Part print with two shaded views. Sizes in mm from the minimum x, y, z corner. Round coordinates to 2 decimals unless told otherwise and drop trailing zeros. Loops run counter-clockwise (first coordinate to the right, second up) from the corner with the lowest first, then second, coordinate; pieces in that order, holes last. Notation, with made-up numbers: (88.5, 24.5) -> (127.5, 24.5) arc R13 ccw to (127.5, 43.5) -> close; hole circle Ø6 at (23, 53). An arc over 180 degrees is marked (long way). Use a Markdown table: item, result. Add a question column.
Item 1: Flat gauge pins, fed straight in: pin 1 (10 mm diameter, centred on y = 6.5, z = 28, fed in from +X); pin 2 (1.5 mm diameter, centred on y = 26.5, z = 34, fed in from +X) (1 decimal). Where does each tip first touch, or does it go through?
Item 2: Cut at C-C, the plane y = 9.5. List the corners of the cut face in (x, z).
Item 3: Cut at D-D, the plane z = 17. List the corners of the cut face in (x, y) (1 decimal).
Item 4: Two-plate mould, pull along X, no slides. Class the marked faces 1, 2 and 3: pulls with the +X half, pulls with the -X half, needs draft (parallel to the pull), parting line crosses it, or undercut.
Item 5: Cut at B-B, the plane x = 23. List the corners of the cut face in (y, z) (1 decimal).
Item 6: Probe line 1 (Z direction, x = 15.5, y = 13); line 2 (X direction, y = 22, z = 22) (1 decimal); line 3 (X direction, y = 8, z = 22). List the from-to ranges inside material, lowest first. Write a range as [from, to].
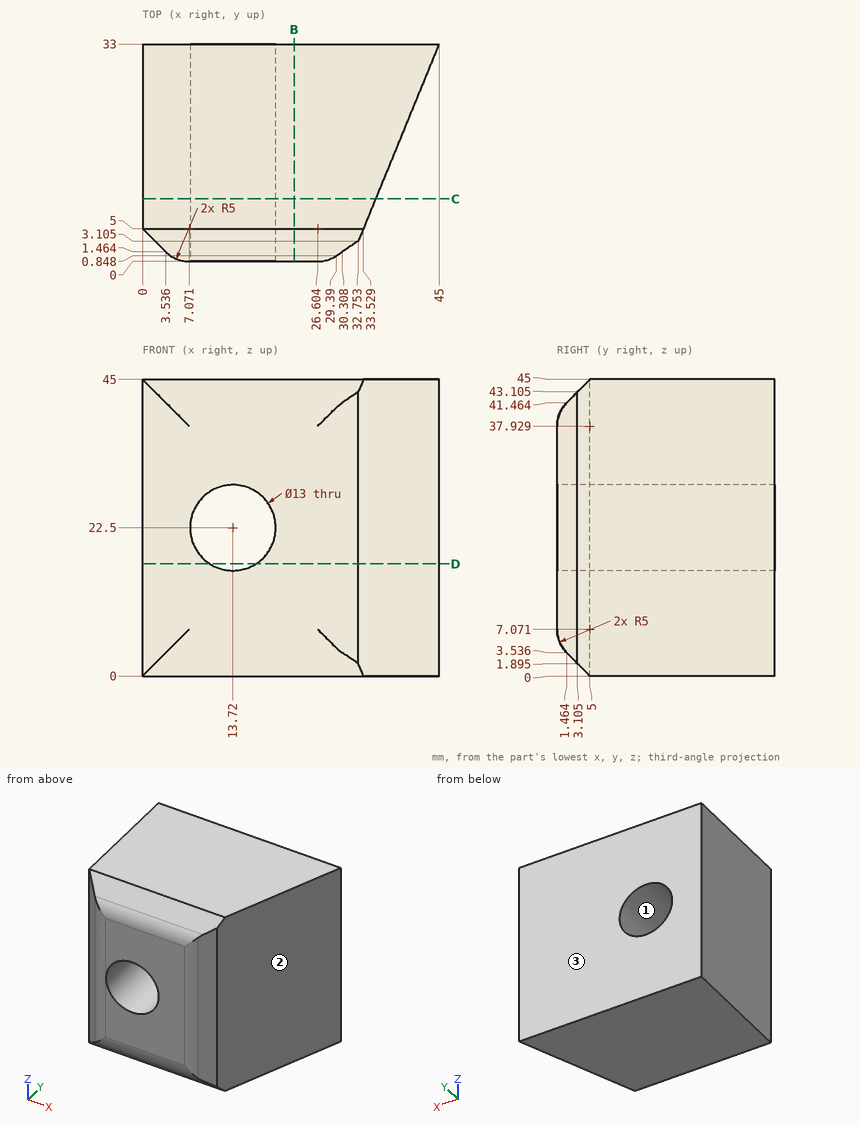
A:
| question | item | result |
|---|---|---|
| 1 | pin 1 | stops at x = 36.19 |
| 1 | pin 2 | stops at x = 42.6 |
| 2 | outline | (0, 0) -> (35.37, 0) -> (35.37, 45) -> (0, 45) -> close; hole circle Ø13 at (13.72, 22.5) |
| 3 | outline | (0, 5) -> (3.5, 1.5) arc R5 ccw to (7.1, 0) -> (10.3, 0) -> (10.3, 33) -> (0, 33) -> close; (17.2, 0) -> (26.6, 0) arc R5 ccw to (29.4, 0.8) -> (32.8, 3.1) -> (45, 33) -> (17.2, 33) -> close |
| 4 | face 1 | undercut |
| 4 | face 2 | pulls with the +X half |
| 4 | face 3 | needs draft |
| 5 | outline | (0, 7.1) arc R5 ccw to (1.5, 3.5) -> (5, 0) -> (33, 0) -> (33, 45) -> (5, 45) -> (1.5, 41.5) arc R5 ccw to (0, 37.9) -> close |
| 6 | line 1 | z = [0, 16.25], [28.75, 45] |
| 6 | line 2 | x = [0, 7.2], [20.2, 40.5] |
| 6 | line 3 | x = [0, 7.24], [20.2, 34.76] |
